Here's how the part is built. I have some questions about the finished solid (model axes, mm). A direction names the side the tool comes from. Coordinates: 2 decimals unless noted, no trailing zeros. Write each loop counter-clockwise with the first axis right and the second up, starting at its lowest first coordinate (ties: lowest second). Pieces come first, ordered by that corner, then holes.
Item 1: I'm going to push a flat-ended pin straight in: P1, Ø1.5, axis at y = 2.5, z = 19.5, coming from the -X side. Where does the tip first touch, or does it pass through?
Item 2: Please list where these lines run through material, in increasing order: line 1 (Y direction, x = 0, z = 52.55); line 2 (Z direction, x = 0, y = 0.3); line 3 (X direction, y = -0.95, z = 52.5).
Item 3: I want a section at D-D (y = 2). Please give me the cut outline in (x, z).
Item 4: I want a section at A-A (x = 0). Please give me the cut outline in (y, z), and give its area (3 significant figures).
Item 5: I want a section at C-C (z = 49). Please give me the cut outline in (x, y), and give its area (3 significant figures).
Item 6: For faces 5 (the face through (1, -1, 0)), 6 (the face through (0, 0, 50)), 7 (the face through (0, 0, 5)), which set-ups out of +Z, -Z, +X, -X, +Y, -Y let a thin tool reach every point of the face, with its end or its side?
Item 7: If we mould it in two halves opening along Y, with no side actions, what happens to faces 1 (the face through (1, -1, 55)), 2 (the face through (-3, 0, 27)), 3 (the face through (-0.27, 1.22, 2.46)), 4 (the face through (-0.27, -1.22, 52.54))? For each: pulls with the +Y half, pulls with the -Y half, needs draft (parallel to the pull), parting line crosses it, or undercut.
Autodesk Inventor part; units mm, degrees
ref_plane "YZ Plane" through (0, 0, 0) normal (1, 0, 0) x (0, 1, 0)
ref_plane "XZ Plane" through (0, 0, 0) normal (0, 1, 0) x (-1, 0, 0)
ref_plane "XY Plane" through (0, 0, 0) normal (0, 0, 1) x (1, 0, 0)
sketch "スケッチ1" plane through (0, 0, 0) normal (0, 0, 1) x (1, 0, 0)
  circle A0 centre (0, 0) radius 3
  circle A1 centre (0, 0) radius 1.25
  dimension "d0" = 6
  dimension "d1" = 2.5
extrude "押し出し1" add sketch "スケッチ1" along normal blind 55 contours A0 | A1
sketch "スケッチ2" plane through (0, 0, 55) normal (0, 0, 1) x (1, 0, 0)
  circle A0 centre (0, 0) radius 3
  circle A1 centre (0, 0) radius 1.25
  dimension "d4" = 2.5
extrude "押し出し2" cut sketch "スケッチ2" against normal blind 5 contours A1
extrude "押し出し3" cut sketch "スケッチ1" along normal blind 5 contours A1
properties part number "50mm" material "アルミニウム 2014-T4"
Answer:
1. P1: stops at x = -2.44
2. line 1: y = -3 to -1.25, 1.25 to 3
2. line 2: z = 5 to 50
2. line 3: x = -2.85 to -0.81, 0.81 to 2.85
3. outline: (-2.24, 0) - (2.24, 0) - (2.24, 55) - (-2.24, 55) - close
4. outline: (-3, 0) - (-1.25, 0) - (-1.25, 5) - (1.25, 5) - (1.25, 0) - (3, 0) - (3, 55) - (1.25, 55) - (1.25, 50) - (-1.25, 50) - (-1.25, 55) - (-3, 55) - close
4. area: 305 mm2
5. outline: circle Ø6 at (0, 0)
5. area: 28.3 mm2
6. face 5: -Z, +X, -X, +Y, -Y
6. face 6: +Z
6. face 7: -Z
7. face 1: needs draft
7. face 2: parting line crosses it
7. face 3: undercut
7. face 4: undercut
